For this review, take the finished solid that the model builds, in its own axes (mm). A direction names the side the tool comes from. Coordinates: 2 decimals unless noted, no trailing zeros. Write each loop counter-clockwise with the first axis right and the second up, starting at its lowest first coordinate (ties: lowest second). Pieces come first, ordered by that corner, then holes. Notation, with made-up numbers: (69.25, 63) -> (94.25, 63) arc R20 cw to (94.25, 75) -> close; hole circle Ø8 at (-20, 60.5). An arc over 180 degrees is marked (long way). One line per item, written item: value. Start each with the question number.
1) Add section D-D (y = -25.75). State the section outline as (x, z) points, and give its area (3 significant figures).
2) For pin 1 Ø8 at (y, z) = (-14, 35.5) entering from -X; pin 2 Ø8 at (x, y) = (40, -13) entering from +Z; pin 3 Ø6 at (x, y) = (67, -21) entering from -Z, all flat-tipped, find the tip position at first contact; note any pin that passes through.
3) Add section A-A (z = 18.5). State the section outline as (x, y) points.
4) Add section B-B (x = 7). State the section outline as (y, z) points, and give its area (3 significant figures).
5) For probe 1 along X at (y, z) = (-12.5, 6); probe 2 along Z at (x, y) = (35, -19.5); probe 3 along X at (y, z) = (-22.5, 25), list the stretches that pass through material, from the lowest coordinate up. Write a range as from..to.
6) Mouldability with a two-part tool opening along X and no side actions: class faces 1 (the flat face through (-51.595, -14, 5)), 2 (the flat face through (0, -10, 22)), 3 (the cylindrical face through (-33.498, -15.575, -2.338)) as released by +X, released by -X, zero draft, split by the parting line, or undercut.
7) Machinability: for faces 4 (the flat face through (-16.283, -14, 28)), 5 (the flat face through (15.517, -20, 22)), 6 (the cylindrical face through (-50.74, -14.15, -22.18)), which of the approach directions +Z, -Z, +X, -X, +Y, -Y give a long, thin tool a straight path to every point of the face, cutting with its end or side? Answer none if there is none.
8) Add section C-C (y = -11.5). State the section outline as (x, z) points, and give its area (3 significant figures).
from build123d import *

# Parameters (mm, degrees)
F1_DEPTH = 27.9
F2_R     = 15
F3_DEPTH = 25
F4_R     = 3
F5_W     = 7.9
F5_H     = 27.016579
F6_DEPTH = 31.8


with BuildPart() as f1:
    # F0 (on Front) → F1 (new body)
    with BuildSketch(Plane.XZ):
        Polygon((15.517242, 43.836206), (-51.594831, 32.586209), (-51.594831, -23.081899), (59.741382, -23.081899), (89.612074, -9.310345), (83.809795, 3.274879), (15.517242, 3.274879), align=None)
    extrude(amount=F1_DEPTH)

    # F2 (on face) → F3 (cut)
    with BuildSketch(Plane.XZ.offset(27.9)):
        with Locations((-21.594828, 6.788793)):
            Circle(F2_R)
    extrude(amount=-F3_DEPTH, mode=Mode.SUBTRACT)

    # F4
    f4_edges = [f1.edges().sort_by_distance(p)[0] for p in [
        (15.517242, -13.95, 43.836206),
        (83.809795, -13.95, 3.274879),
        (89.612074, -13.95, -9.310345),
        (59.741382, -13.95, -23.081899),
        (-51.594831, -13.95, -23.081899),
        (-51.594831, -13.95, 32.586209),
    ]]
    fillet(f4_edges, radius=F4_R)

    # F5 (on face) → F6 (cut)
    with BuildSketch(Plane.YZ.offset(15.517242)):
        with Locations((-13.95, 21.783168)):
            Rectangle(F5_W, F5_H)
    extrude(amount=-F6_DEPTH, mode=Mode.SUBTRACT)


solid = f1.part
Numbers:
1. outline: (-51.59, -20.08) arc R3 ccw to (-48.59, -23.08) -> (59.08, -23.08) arc R3 ccw to (60.34, -22.81) -> (86.89, -10.57) arc R3 ccw to (88.36, -6.59) -> (84.61, 1.53) arc R3 ccw to (81.89, 3.27) -> (15.52, 3.27) -> (15.52, 40.29) arc R3 ccw to (12.02, 43.25) -> (-49.09, 33.01) arc R3 ccw to (-51.59, 30.05) -> close; hole circle Ø30 at (-21.59, 6.79)
1. area: 5,110 mm²
2. pin 1: x = -51.22
2. pin 2: z = 3.27
2. pin 3: z = -21.12
3. outline: (-51.59, -27.9) -> (-30.97, -27.9) -> (-30.97, -2.9) -> (-12.22, -2.9) -> (-12.22, -10) -> (15.52, -10) -> (15.52, 0) -> (-51.59, 0) -> close; (-12.22, -27.9) -> (15.52, -27.9) -> (15.52, -17.9) -> (-12.22, -17.9) -> close
4. outline: (-27.9, -23.08) -> (0, -23.08) -> (0, 42.41) -> (-27.9, 42.41) -> close; hole (-17.9, 8.27) -> (-10, 8.27) -> (-10, 35.29) -> (-17.9, 35.29) -> close
4. area: 1,610 mm²
5. probe 1: -51.59..-36.57, -6.62..15.52
5. probe 2: -23.08..3.27
5. probe 3: -51.59..15.52
6. face 1: released by -X
6. face 2: zero draft
6. face 3: undercut
7. face 4: +X
7. face 5: +Z, +X, +Y, -Y
7. face 6: -Z, -X, +Y, -Y
8. outline: (-51.59, -20.08) arc R3 ccw to (-48.59, -23.08) -> (59.08, -23.08) arc R3 ccw to (60.34, -22.81) -> (86.89, -10.57) arc R3 ccw to (88.36, -6.59) -> (84.61, 1.53) arc R3 ccw to (81.89, 3.27) -> (15.52, 3.27) -> (15.52, 8.27) -> (-6.67, 8.27) arc R15 cw (long way) to (-16.28, 20.82) -> (-16.28, 35.29) -> (15.52, 35.29) -> (15.52, 40.29) arc R3 ccw to (12.02, 43.25) -> (-49.09, 33.01) arc R3 ccw to (-51.59, 30.05) -> close
8. area: 4,330 mm²
